from build123d import *

# Parameters (mm, degrees)
SKETCH1_R           = 1.5
SKETCH1_R_2         = 5
BOSS_EXTRUDE1_DEPTH = 3


with BuildPart() as part:
    # Sketch1 → Boss-Extrude1 (new body)
    with BuildSketch(Plane(origin=(0, 0, 0), x_dir=(1, 0, 0), z_dir=(0, 1, 0))):
        with BuildLine():
            Line((-15, 21.693547428), (-15, 38.108016468))
            ThreePointArc((-15, 38.108016468), (-14.121320344, 40.229336812), (-12, 41.108016468))
            Line((-12, 41.108016468), (12, 41.108016468))
            ThreePointArc((12, 41.108016468), (14.121320344, 40.229336812), (15, 38.108016468))
            Line((15, 38.108016468), (15, 21.693547428))
            ThreePointArc((15, 21.693547428), (15.631737063, 18.195598093), (17.447129909, 15.139605607))
            ThreePointArc((17.447129909, 15.139605607), (23.1, 0), (17.447129909, -15.139605607))
            ThreePointArc((17.447129909, -15.139605607), (15.631737063, -18.195598093), (15, -21.693547428))
            Line((15, -21.693547428), (15, -38.108016468))
            ThreePointArc((15, -38.108016468), (14.121320344, -40.229336812), (12, -41.108016468))
            Line((12, -41.108016468), (-12, -41.108016468))
            ThreePointArc((-12, -41.108016468), (-14.121320344, -40.229336812), (-15, -38.108016468))
            Line((-15, -38.108016468), (-15, -21.693547428))
            ThreePointArc((-15, -21.693547428), (-15.631737063, -18.195598093), (-17.447129909, -15.139605607))
            ThreePointArc((-17.447129909, -15.139605607), (-23.1, 0), (-17.447129909, 15.139605607))
            ThreePointArc((-17.447129909, 15.139605607), (-15.631737063, 18.195598093), (-15, 21.693547428))
        make_face()
        with Locations(Location((-8.838834765, 8.838834765, 0), (0, 0, 270))):
            Circle(SKETCH1_R, mode=Mode.SUBTRACT)
        with Locations(Location((8.838834765, -8.838834765, 0), (0, 0, 90))):
            Circle(SKETCH1_R, mode=Mode.SUBTRACT)
        with Locations(Location((6.717514421, 6.717514421, 0), (0, 0, 270))):
            Circle(SKETCH1_R, mode=Mode.SUBTRACT)
        with Locations(Location((-6.717514421, -6.717514421, 0), (0, 0, 90))):
            Circle(SKETCH1_R, mode=Mode.SUBTRACT)
        with Locations(Location((0, 0, 0), (0, 0, 270))):
            Circle(SKETCH1_R_2, mode=Mode.SUBTRACT)
        with Locations(Location((-8.838834765, 33.462792438, 0), (0, 0, 270))):
            Circle(SKETCH1_R, mode=Mode.SUBTRACT)
        with Locations(Location((8.838834765, 33.462792438, 0), (0, 0, 90))):
            Circle(SKETCH1_R, mode=Mode.SUBTRACT)
        with Locations(Location((8.838834765, -33.462792438, 0), (0, 0, 270))):
            Circle(SKETCH1_R, mode=Mode.SUBTRACT)
        with Locations(Location((-8.838834765, -33.462792438, 0), (0, 0, 90))):
            Circle(SKETCH1_R, mode=Mode.SUBTRACT)
    extrude(amount=BOSS_EXTRUDE1_DEPTH)


solid = part.part
Part model, mm, in its own coordinate system. A direction names the side the tool comes from. Round coordinates to 2 decimals unless told otherwise and drop trailing zeros. Write each loop counter-clockwise with the first axis right and the second up, starting at its lowest first coordinate (ties: lowest second). Pieces come first, ordered by that corner, then holes. Notation, with made-up numbers: M -19,49 L 19,49 A17 cw 19,53 Z; hole C 51.5,-39.75 d10. An arc over 180 degrees is marked long. Return JSON: item names as keys, results as strings. Group by question number.
(1) Saw through at C-C on y = 0.65. Count the separate pieces of the cut face and the enclosed holes in it, then the cut area to 3 significant figures.
(2) Saw through at D-D on z = -28. Write the cut outline in (x, y), then the cut area to 3 significant figures.
(3) Drill centre lines: probe 1 along X at (y, z) = (1.05, -30); probe 2 along Z at (x, y) = (-8.5, 2.6); probe 3 along Z at (x, y) = (2, 1.95). Where is each one in solid material? Low to high.
(4) Pin check, flat tips, straight feed: pin 1 Ø1.5 at (y, z) = (1, 30) entering from +X; pin 2 Ø1 at (y, z) = (1.5, -3) entering from +X. Stop position of each tip, or through.
(5) Two-plate mould, pull along X, no slides. Class faces 4 (the face through (-9.75, 1.48, -10.03)), 5 (the face through (-14.1, 1.48, 40.25)), 6 (the face through (5.5, 3, -0.6)), 7 (the face through (23.1, 1.5, -0.2)): +X half, -X half, draft (parallel to the pull), parting line (faces both ways), or undercut.
(6) Saw through at B-B on x = 0. Write the cut outline in (y, z).
(7) Which spindle directions (+Z, -Z, +X, -X, +Y, -Y) get a long thin tool onto all of the face, cutting with end or side? Do faces 1 (the face through (-15, 1, -30)), 2 (the face through (15, 1, -30)), 3 (the face through (-15, 1, 30)). Say none if no direction does.
(8) Saw through at A-A on z = 0. Write the cut outline in (x, y), then the cut area to 3 significant figures.
Returned:
{
 "1": {"separate pieces": "1", "enclosed holes": "9", "area": "2,730 mm²"},
 "2": {"outline": "M -15,0 L 15,0 L 15,3 L -15,3 Z", "area": "90.0 mm²"},
 "3": {"probe 1": "-15 to 15", "probe 2": "-41.11 to -34.92, -32 to -10.3, -7.38 to 32, 34.92 to 41.11", "probe 3": "-41.11 to -4.58, 4.58 to 41.11"},
 "4": {"pin 1": "x = 15", "pin 2": "x = 22.96"},
 "5": {"face 4": "undercut", "face 5": "-X half", "face 6": "draft", "face 7": "+X half"},
 "6": {"outline": "M 0,-41.11 L 3,-41.11 L 3,-5 L 0,-5 Z; M 0,5 L 3,5 L 3,41.11 L 0,41.11 Z"},
 "7": {"face 1": "-Z, -X, +Y, -Y", "face 2": "-Z, +X, +Y, -Y", "face 3": "+Z, -X, +Y, -Y"},
 "8": {"outline": "M -23.1,0 L -5,0 L -5,3 L -23.1,3 Z; M 5,0 L 23.1,0 L 23.1,3 L 5,3 Z", "area": "109 mm²"}
}
